from build123d import *

# Parameters (mm, degrees)
SKETCH1_R             = 1.275
BOSS_EXTRUDE1_DEPTH   = 6.5
SKETCH3_W             = 3.2
SKETCH3_H             = 0.56
SKETCH3_H_2           = 0.5
BOSS_EXTRUDE3_DEPTH   = 0.9
SKETCH4_W             = 1.2
SKETCH4_H             = 0.56
SKETCH4_H_2           = 0.5
BOSS_EXTRUDE4_DEPTH   = 3.47
FILLET2_R             = 0.59
ESBO_O1_R             = 0.1
CORTE_EXTRUS_O1_DEPTH = 40.747314551


with BuildPart() as part:
    # Sketch1 → Boss-Extrude1 (new body)
    with BuildSketch(Plane(origin=(0, 0, 0), x_dir=(0, 0, -1), z_dir=(1, 0, 0))):
        with BuildLine():
            Line((-37.373122581, 0), (-34.673122581, 0))
            Line((-34.673122581, 0), (-34.673122581, -0.45))
            Line((-34.673122581, -0.45), (-30.873122581, -0.45))
            Line((-30.873122581, -0.45), (-30.873122581, 0))
            Line((-30.873122581, 0), (-24.973122581, 0))
            Line((-24.973122581, 0), (-24.973122581, -0.45))
            Line((-24.973122581, -0.45), (-21.173122581, -0.45))
            Line((-21.173122581, -0.45), (-21.173122581, 0))
            Line((-21.173122581, 0), (-18.673122581, 0))
            ThreePointArc((-18.673122581, 0), (-18.31956919, 0.146446609), (-18.173122581, 0.5))
            Line((-18.173122581, 0.5), (-18.173122581, 9.02))
            ThreePointArc((-18.173122581, 9.02), (-18.31956919, 9.373553391), (-18.673122581, 9.52))
            Line((-18.673122581, 9.52), (-28.173122581, 9.52))
            Line((-28.173122581, 9.52), (-28.173122581, 10.16))
            Line((-28.173122581, 10.16), (-37.373122581, 10.16))
            ThreePointArc((-37.373122581, 10.16), (-37.726675972, 10.013553391), (-37.873122581, 9.66))
            Line((-37.873122581, 9.66), (-37.873122581, 0.5))
            ThreePointArc((-37.873122581, 0.5), (-37.726675972, 0.146446609), (-37.373122581, 0))
        make_face()
        with Locations(Location((-32.773122581, 2.525, 0), (0, 0, 180))):
            Circle(SKETCH1_R, mode=Mode.SUBTRACT)
        with Locations(Location((-23.073122581, 2.525, 0), (0, 0, 180))):
            Circle(SKETCH1_R, mode=Mode.SUBTRACT)
    extrude(amount=BOSS_EXTRUDE1_DEPTH)

    # Sketch3 → Boss-Extrude3 (add)
    with BuildSketch(Plane(origin=(0, 0, 0), x_dir=(-1, 0, 0), z_dir=(0, -1, 0))):
        with Locations((-3.25, -36.193122581)):
            Rectangle(SKETCH3_W, SKETCH3_H)
        with Locations((-3.25, -27.223122581)):
            Rectangle(SKETCH3_W, SKETCH3_H_2)
        with Locations((-3.25, -20.023122581)):
            Rectangle(SKETCH3_W, SKETCH3_H_2)
    extrude(amount=BOSS_EXTRUDE3_DEPTH)

    # Sketch4 → Boss-Extrude4 (add)
    with BuildSketch(Plane(origin=(0, -0.9, 0), x_dir=(-1, 0, 0), z_dir=(0, -1, 0))):
        with Locations((-3.25, -36.193122581)):
            Rectangle(SKETCH4_W, SKETCH4_H)
        with Locations((-3.25, -27.223122581)):
            Rectangle(SKETCH4_W, SKETCH4_H_2)
        with Locations((-3.25, -20.023122581)):
            Rectangle(SKETCH4_W, SKETCH4_H_2)
    extrude(amount=BOSS_EXTRUDE4_DEPTH)

    # Fillet2
    fillet2_edges = [part.edges().sort_by_distance(p)[0] for p in [
        (2.65, -4.37, 36.193122581),
        (3.85, -4.37, 36.193122581),
        (2.65, -4.37, 27.223122581),
        (3.85, -4.37, 27.223122581),
        (3.85, -4.37, 20.023122581),
        (2.65, -4.37, 20.023122581),
    ]]
    fillet(fillet2_edges, radius=FILLET2_R)

    # Esboço1 → Corte-extrusão1 (cut, through all)
    with BuildSketch(Plane.ZY):
        with Locations((34.873122581, 10.16)):
            Circle(ESBO_O1_R)
    extrude(amount=-CORTE_EXTRUS_O1_DEPTH, mode=Mode.SUBTRACT)


solid = part.part
Verification items for the finished model (mm, model axes). A direction names the side the tool comes from. Coordinates: 2 decimals unless noted, no trailing zeros. Order: outer loops, then holes, each group sorted by start corner. A loop starts at its lowest first (then second) coordinate and runs counter-clockwise, first axis right, second up. Notation, with made-up numbers: M 57,-25.75 L 79,-25.75 A15 ccw 79,-7.75 Z; hole C 12.5,10 d2. An arc over 180 degrees is marked long. Write each question's results on one line, items separated by ' | '.
1) Section check A-A on y = -3.25. Record the cut outline in (x, z), plus the area to 3 significant figures.
Solved:
outline: M 2.65,19.77 L 3.85,19.77 L 3.85,20.27 L 2.65,20.27 Z; M 2.65,26.97 L 3.85,26.97 L 3.85,27.47 L 2.65,27.47 Z; M 2.65,35.91 L 3.85,35.91 L 3.85,36.47 L 2.65,36.47 Z | area: 1.87 mm²
2) Section check C-C on x = 6. Record the cut outline in (y, z) (3 decimals), plus the area to 3 significant figures.
Solved:
outline: M -0.45,21.173 L 0,21.173 L 0,18.673 A0.5 ccw 0.5,18.173 L 9.02,18.173 A0.5 ccw 9.52,18.673 L 9.52,28.173 L 10.16,28.173 L 10.16,34.773 A0.1 cw 10.16,34.973 L 10.16,37.373 A0.5 ccw 9.66,37.873 L 0.5,37.873 A0.5 ccw 0,37.373 L 0,34.673 L -0.45,34.673 L -0.45,30.873 L 0,30.873 L 0,24.973 L -0.45,24.973 Z; hole C 2.525,23.073 d2.55; hole C 2.525,32.773 d2.55 | area: 187 mm²
3) Access from +Z, -Z, +X, -X, +Y, -Y to the whole of each face (thin tool, end or side, straight path). Record for faces 1 (the face through (3, -0.45, 23)), 2 (the face through (3, -2, 19.773)), 3 (the face through (3, 9.52, 23)), 4 (the face through (3, 5, 18.173)).
Solved:
face 1: +X, -X, -Y | face 2: -Z, +X, -X, -Y | face 3: -Z, +X, -X, +Y | face 4: -Z, +X, -X, +Y, -Y
4) Gauge pin test, flat ends, axial feed: pin 1 Ø1 at (x, y) = (4, -1) entering from -Z; pin 2 Ø1.6 at (x, y) = (4, -2.5) entering from +Z; pin 3 Ø0.6 at (x, z) = (2, 36) entering from -Y. Record the tip position at first contact, or that the pin passes through.
Solved:
pin 1: stops at z = 19.77 | pin 2: stops at z = 36.47 | pin 3: stops at y = -0.9
5) Release check for a two-part mould opening along Y. For faces 5 (the face through (3, -2, 35.913)), 6 (the face through (3.2, 2.5, 31.5)), 7 (the face through (3, 10.16, 36)) record: pulls with the +Y half, pulls with the -Y half, needs draft (parallel to the pull), parting line crosses it, or undercut.
Solved:
face 5: needs draft | face 6: undercut | face 7: pulls with the +Y half
6) Scan lines: line 1 along Z through (x, y) = (3.5, -3.75); line 2 along Z through (x, y) = (6, 1.75); line 3 along Y through (x, z) = (5.5, 36). Record each from-to range of solid material in increasing order. Write a range as [from, to].
Solved:
line 1: z = [19.77, 20.27], [26.97, 27.47], [35.91, 36.47] | line 2: z = [18.17, 22.06], [24.09, 31.76], [33.79, 37.87] | line 3: y = [0, 10.16]
7) Section check B-B on z = 22.75. Record the cut outline in (x, y).
Solved:
outline: M 0,-0.45 L 6.5,-0.45 L 6.5,1.29 L 0,1.29 Z; M 0,3.76 L 6.5,3.76 L 6.5,9.52 L 0,9.52 Z
8) Section check D-D on z = 29. Record the cut outline in (x, y), plus the area to 3 significant figures.
Solved:
outline: M 0,0 L 6.5,0 L 6.5,10.16 L 0,10.16 Z | area: 66.0 mm²
